The figure shows three views and two pictorial views of one solid part (mm, origin at its lowest corner). Answer the questions. Give positions to 0.01 mm unless a question says otherwise; leave off trailing zeros. Loops run counter-clockwise (first coordinate to the right, second up) from the corner with the lowest first, then second, coordinate; pieces in that order, holes last. Notation, with made-up numbers: (-9, 12.5) - (19, 12.5) arc R34 cw to (19, 48.5) - close; hole circle Ø8 at (80.25, 79). An arc over 180 degrees is marked (long way). Write each question's results on one line, items separated by ' | '.
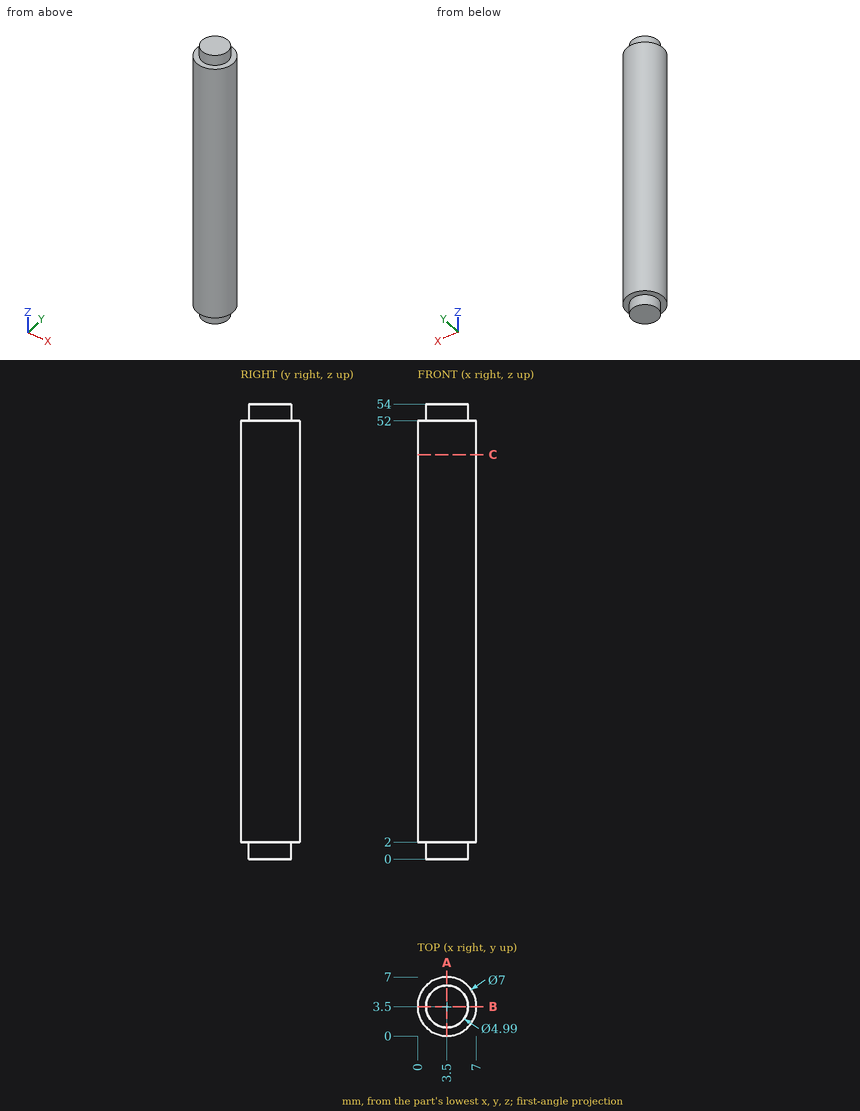
Item 1: Flat-ended cylindrical pins translate along their axes: P1, Ø2, axis at y = 6, z = 18, coming from the -X side; P2, Ø1.5, axis at x = 5.5, z = 10, coming from the +Y side; P3, Ø3, axis at y = 6, z = 14, coming from the +X side. Find the tip coordinate at first contact, or state that the pin passes through.
Values found:
P1: stops at x = 0.34 | P2: stops at y = 6.77 | P3: stops at x = 6.85
Item 2: A cutting plane is placed at C-C, the plane z = 48. Determine the outline of the cut face in (x, y), plus the area to 3 significant figures.
Values found:
outline: circle Ø7 at (3.5, 3.5) | area: 38.5 mm²
Item 3: Find the intervals of material crossed by line 1 along Z through (x, y) = (5.5, 1.5); line 2 along Y through (x, z) = (3.25, 50.5), in increasing order. Write a range as [from, to].
Values found:
line 1: z = [2, 52] | line 2: y = [0.01, 6.99]
Item 4: A cutting plane is placed at A-A, the plane x = 3.5. Determine the outline of the cut face in (y, z) (3 decimals).
Values found:
outline: (0, 2) - (1.005, 2) - (1.005, 0) - (5.995, 0) - (5.995, 2) - (7, 2) - (7, 52) - (5.995, 52) - (5.995, 54) - (1.005, 54) - (1.005, 52) - (0, 52) - close
